The listing builds one solid part. Answer for the finished solid, in the listing's coordinates (mm). Face numbers are marked on the shaded views. A direction names the side the tool comes from. Give positions to 0.01 mm unless a question says otherwise; leave off trailing zeros. Order: outer loops, then holes, each group sorted by start corner. A loop starts at its lowest first (then second) coordinate and runs counter-clockwise, first axis right, second up. Notation, with made-up numbers: (46, -34) - (58, -34) arc R25 cw to (58, 5) - close; hole circle Ø5 at (18.5, 21.25). An arc over 180 degrees is marked (long way). Use a Markdown table: item, result. Add a question column.
1) Find section C-C, the plane y = 4. Determine the outline of the cut face in (x, z), plus the area to 3 significant figures.
2) Find section D-D, the plane x = -0.25. Determine the outline of the cut face in (y, z), plus the area to 3 significant figures.
3) Find section B-B, the plane y = -2. Determine the outline of the cut face in (x, z), plus the area to 3 significant figures.
4) Flat-ended cylindrical pins translate along their axes: pin 1 (3 mm diameter, centred on y = 1, z = 10, fed in from -X); pin 2 (3.5 mm diameter, centred on y = -5, z = 8.5, fed in from -X); pin 3 (1 mm diameter, centred on x = -3.5, y = -2.5, fed in from +Z). Find the tip coordinate at first contact, or state that the pin passes through.
5) For the marked faces 4, 5 and 6, determine the directions among +Z, -Z, +X, -X, +Y, -Y from which every point of the face is accessible in a straight line to the end or side of a thin tool.
6) Straight lines are drawn through the part: line 1 (X direction, y = 0, z = 2.45); line 2 (Y direction, x = 0, z = 1.25); line 3 (Y direction, x = 4.1, z = 8.5). For each, find the intervals that lie inside material, in ascending order.
7) The mould has two halves that part along Y. Classify the marked faces 1, 2 and 3: released by +Y, released by -Y, zero draft, split by the parting line, or undercut.
8) Find section A-A, the plane z = 8.5. Determine the outline of the cut face in (x, y).
from build123d import *
from build123d.topology import SkipClean

# Parameters (mm, degrees)
SKETCH_1_W          = 12
SKETCH_1_H          = 12
SKETCH_1_R          = 3
EXTRUDE_1_DEPTH     = 5
EXTRUDE_2_DEPTH     = 7
SKETCH_4_R          = 1.75
CUT_EXTRUDE_1_DEPTH = 7
SKETCH_5_R          = 3.5
CUT_EXTRUDE_2_DEPTH = 3
FILLET_1_R          = 2
FILLET_2_R          = 1.5
FILLET_3_R          = 2
SKETCH_6_W          = 51.167953154
SKETCH_6_H          = 21.993207172
CUT_EXTRUDE_3_DEPTH = 1


with BuildPart() as part:
    # 草图1 → 凸台-拉伸1 (new body)
    with BuildSketch(Plane.XY):
        Rectangle(SKETCH_1_W, SKETCH_1_H)
        Circle(SKETCH_1_R, mode=Mode.SUBTRACT)
    extrude(amount=EXTRUDE_1_DEPTH)

    # 草图3 → 凸台-拉伸2 (add)
    with BuildSketch(Plane.XY.offset(5)):
        with BuildLine():
            Line((0, -6), (6, -6))
            Line((6, -6), (6, 6))
            Line((6, 6), (0, 6))
            Line((0, 6), (0, 3))
            ThreePointArc((0, 3), (3, 0), (0, -3))
            Line((0, -3), (0, -6))
        make_face()
    extrude(amount=EXTRUDE_2_DEPTH)

    # 草图4 → 切除-拉伸1 (cut)
    with BuildSketch(Plane.ZY):
        with Locations((8.5, 0)):
            Circle(SKETCH_4_R)
    extrude(amount=-CUT_EXTRUDE_1_DEPTH, mode=Mode.SUBTRACT)

    # 草图5 → 切除-拉伸2 (cut)
    with SkipClean():  # the faces are left unmerged after this step: merging them gives an invalid solid
        with BuildSketch(Plane.ZY):
            with Locations((8.5, 0)):
                Circle(SKETCH_5_R)
        extrude(amount=-CUT_EXTRUDE_2_DEPTH, mode=Mode.SUBTRACT)

    # 圆角1
    # the kernel refuses this fillet: 2 mm, written as the material it adds along each edge
    with BuildSketch(Plane(origin=(0, 2, 5), x_dir=(-1, 0, 0), z_dir=(0, -1, 0))) as fillet_1_piece_1_section:
        with BuildLine():
            CenterArc((FILLET_1_R, -FILLET_1_R), FILLET_1_R, 90, 90)
            Line((0, -FILLET_1_R), (0, 0))
            Line((0, 0), (FILLET_1_R, 0))
        make_face()
    fillet_1_piece_1 = extrude(amount=8, mode=Mode.PRIVATE)
    fillet_1_piece_1 = fillet_1_piece_1 - Plane(origin=(0, 0, 5), x_dir=(1, 0, 0), z_dir=(0, 0, -1)) * Cylinder(3, 24, mode=Mode.PRIVATE)
    fillet_1_piece_1 = fillet_1_piece_1 - Plane(origin=(0, 0, 8.5), x_dir=(0, 0, 1), z_dir=(-1, 0, 0)) * Cylinder(3.5, 24, mode=Mode.PRIVATE)
    add(fillet_1_piece_1)
    with BuildSketch(Plane(origin=(0, 6, 5), x_dir=(-1, 0, 0), z_dir=(0, -1, 0))) as fillet_1_piece_2_section:
        with BuildLine():
            CenterArc((FILLET_1_R, -FILLET_1_R), FILLET_1_R, 90, 90)
            Line((0, -FILLET_1_R), (0, 0))
            Line((0, 0), (FILLET_1_R, 0))
        make_face()
    fillet_1_piece_2 = extrude(amount=8, mode=Mode.PRIVATE)
    fillet_1_piece_2 = fillet_1_piece_2 - Plane(origin=(0, 0, 5), x_dir=(1, 0, 0), z_dir=(0, 0, -1)) * Cylinder(3, 24, mode=Mode.PRIVATE)
    fillet_1_piece_2 = fillet_1_piece_2 - Plane(origin=(0, 0, 8.5), x_dir=(0, 0, 1), z_dir=(-1, 0, 0)) * Cylinder(3.5, 24, mode=Mode.PRIVATE)
    add(fillet_1_piece_2)

    # 圆角2
    fillet_2_edges = [part.edges().sort_by_distance(p)[0] for p in [
        (3, 6, 12),
        (3, -6, 12),
    ]]
    fillet(fillet_2_edges, radius=FILLET_2_R)

    # 圆角3
    fillet_3_edges = [part.edges().sort_by_distance(p)[0] for p in [
        (-6, 0, 5),
    ]]
    fillet(fillet_3_edges, radius=FILLET_3_R)

    # 草图6 → 切除-拉伸3 (cut)
    with BuildSketch(Plane(origin=(6, 0, 0), x_dir=(0, 0, -1), z_dir=(1, 0, 0))):
        with Locations((-8.5, 0)):
            Rectangle(SKETCH_6_W, SKETCH_6_H)
    extrude(amount=-CUT_EXTRUDE_3_DEPTH, mode=Mode.SUBTRACT)


solid = part.part
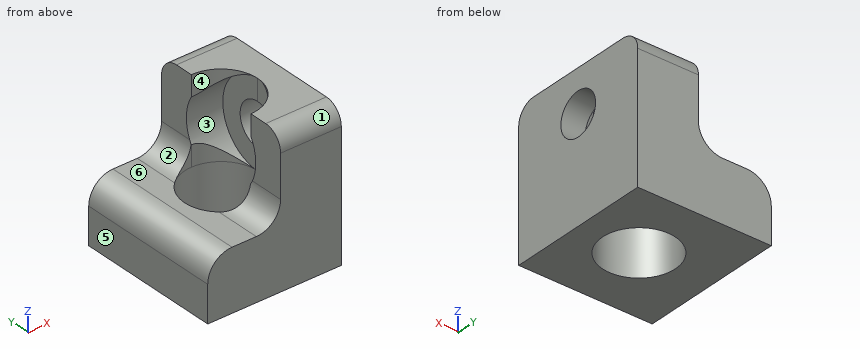
The answers:
| question | item | result |
|---|---|---|
| 1 | outline | (-6, 0) - (5, 0) - (5, 12) - (0, 12) - (0, 7) arc R2 cw to (-2, 5) - (-4, 5) arc R2 ccw to (-6, 3) - close |
| 1 | area | 90.0 mm2 |
| 2 | outline | (-6, 0) - (-2.99, 0) - (-2.99, 6.03) - (-6, 6.03) - close; (2.99, 0) - (6, 0) - (6, 6.03) - (2.99, 6.03) - close |
| 2 | area | 36.3 mm2 |
| 3 | outline | (-6, 0) - (-2.24, 0) - (-2.24, 5) - (-4, 5) arc R2 ccw to (-6, 3) - close; (2.24, 0) - (5, 0) - (5, 12) - (2.24, 12) - (2.24, 11.37) - (3, 11.37) - (3, 5.63) - (2.24, 5.63) - close |
| 3 | area | 46.7 mm2 |
| 4 | pin 1 | x = 3 |
| 4 | pin 2 | x = -0.02 |
| 4 | pin 3 | z = 5 |
| 5 | face 4 | +Z, -Z, -X |
| 5 | face 5 | +Z, -Z, -X, +Y, -Y |
| 5 | face 6 | +Z, -X, +Y, -Y |
| 6 | line 1 | -6 to -3, 3 to 5 |
| 6 | line 2 | -6 to -3, 3 to 6 |
| 6 | line 3 | -6 to -1.75, 1.75 to 6 |
| 7 | face 1 | released by -Y |
| 7 | face 2 | zero draft |
| 7 | face 3 | undercut |
| 8 | outline | (0, -6) - (5, -6) - (5, -1.75) - (3, -1.75) - (3, -3.5) - (0, -3.5) - close; (0, 3.5) - (3, 3.5) - (3, 1.75) - (5, 1.75) - (5, 6) - (0, 6) - close |
